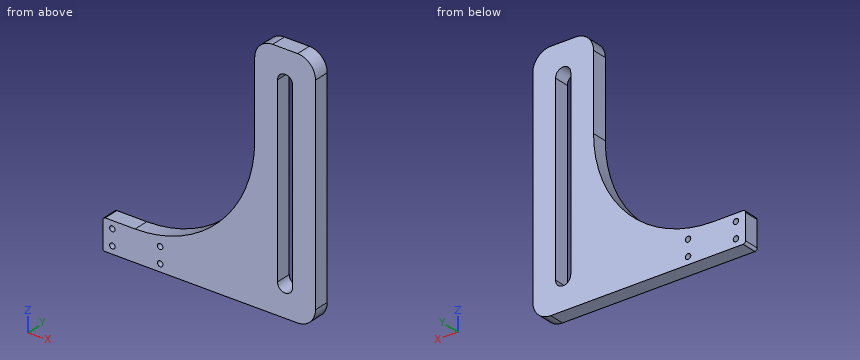
```python
from build123d import *

# Parameters (mm, degrees)
SKETCH1_R           = 1.1303
BOSS_EXTRUDE2_DEPTH = 6.35
FILLET1_R           = 1
FILLET2_R           = 7.5


with BuildPart() as part:
    # Sketch1 → Boss-Extrude2 (new body)
    with BuildSketch(Plane(origin=(0, 0, 0), x_dir=(1, 0, 0), z_dir=(0, 1, 0))):
        with BuildLine():
            Line((-12.7, 50.8), (-76.2, 50.8))
            Line((-76.2, 50.8), (-76.2, 38.1))
            Line((-76.2, 38.1), (-62.7, 38.1))
            ThreePointArc((-62.7, 38.1), (-27.344660941, 23.455339059), (-12.7, -11.9))
            Line((-12.7, -11.9), (-12.7, -50.8))
            Line((-12.7, -50.8), (12.7, -50.8))
            Line((12.7, -50.8), (12.7, 50.8))
            Line((12.7, 50.8), (-12.7, 50.8))
        make_face()
        with Locations(Location((-72.2, 47.7, 0), (0, 0, 270))):
            Circle(SKETCH1_R, mode=Mode.SUBTRACT)
        with Locations(Location((-72.2, 41.2, 0), (0, 0, 270))):
            Circle(SKETCH1_R, mode=Mode.SUBTRACT)
        with Locations(Location((-52.2, 47.7, 0), (0, 0, 270))):
            Circle(SKETCH1_R, mode=Mode.SUBTRACT)
        with Locations(Location((-52.2, 41.2, 0), (0, 0, 270))):
            Circle(SKETCH1_R, mode=Mode.SUBTRACT)
        with BuildLine():
            Line((-3.175, -38.1), (-3.175, 38.1))
            ThreePointArc((-3.175, 38.1), (0, 41.275), (3.175, 38.1))
            Line((3.175, 38.1), (3.175, -38.1))
            ThreePointArc((3.175, -38.1), (0, -41.275), (-3.175, -38.1))
        make_face(mode=Mode.SUBTRACT)
    extrude(amount=BOSS_EXTRUDE2_DEPTH)

    # Fillet1
    fillet1_edges = [part.edges().sort_by_distance(p)[0] for p in [
        (-76.2, 3.175, -38.1),
        (-76.2, 3.175, -50.8),
    ]]
    fillet(fillet1_edges, radius=FILLET1_R)

    # Fillet2
    fillet2_edges = [part.edges().sort_by_distance(p)[0] for p in [
        (12.7, 3.175, 50.8),
        (-12.7, 3.175, 50.8),
        (12.7, 3.175, -50.8),
    ]]
    fillet(fillet2_edges, radius=FILLET2_R)


solid = part.part
```
Model file for the job. Use its own axes, mm. Give positions to 0.01 mm unless a question says otherwise; leave off trailing zeros. Order: outer loops, then holes, each group sorted by start corner. A loop starts at its lowest first (then second) coordinate and runs counter-clockwise, first axis right, second up.
1) Pin check, flat tips, straight feed: pin 1 (1.5 mm diameter, centred on x = -30.5, y = 3, fed in from +Z); pin 2 (1.9 mm diameter, centred on y = 2, z = -7, fed in from -X); pin 3 (2 mm diameter, centred on y = 3, z = 22.5, fed in from -X). Stop position of each tip, or through.
2) Saw through at B-B, the plane x = -52.2. Write the cut outline in (y, z), then the cut area to 3 significant figures.
3) Wall check: probe 1 along Z at (x, y) = (-72.2, 5); probe 2 along X at (y, z) = (3, 33) (3 decimals); probe 3 along Z at (x, y) = (-52, 5). Give the ranges that are in metal, low to high.
4) Saw through at C-C, the plane y = 2. Write the cut outline in (x, z) (3 decimals), then the cut area to 3 significant figures.
5) Saw through at A-A, the plane z = -22. Write the cut outline in (x, y) (3 decimals), then the cut area to 3 significant figures.
6) Saw through at D-D, the plane z = -47.7. Write the cut outline in (x, y).
Computed:
1. pin 1: stops at z = -25.71
1. pin 2: stops at x = -16.81
1. pin 3: stops at x = -12.7
2. outline: (0, -50.8) - (6.35, -50.8) - (6.35, -48.83) - (0, -48.83) - close; (0, -46.57) - (6.35, -46.57) - (6.35, -42.33) - (0, -42.33) - close; (0, -40.07) - (6.35, -40.07) - (6.35, -36.99) - (0, -36.99) - close
2. area: 59.0 mm2
3. probe 1: z = -50.8 to -48.83, -46.57 to -42.33, -40.07 to -38.1
3. probe 2: x = -12.7 to -3.175, 3.175 to 12.7
3. probe 3: z = -50.8 to -48.81, -46.59 to -42.31, -40.09 to -36.94
4. outline: (-76.2, -49.8) arc R1 ccw to (-75.2, -50.8) - (5.2, -50.8) arc R7.5 ccw to (12.7, -43.3) - (12.7, 43.3) arc R7.5 ccw to (5.2, 50.8) - (-5.2, 50.8) arc R7.5 ccw to (-12.7, 43.3) - (-12.7, 11.9) arc R50 cw to (-62.7, -38.1) - (-75.2, -38.1) arc R1 ccw to (-76.2, -39.1) - close; hole circle Ø2.261 at (-72.2, -47.7); hole circle Ø2.261 at (-72.2, -41.2); hole circle Ø2.261 at (-52.2, -47.7); hole circle Ø2.261 at (-52.2, -41.2); hole (-3.175, -38.1) arc R3.175 ccw to (3.175, -38.1) - (3.175, 38.1) arc R3.175 ccw to (-3.175, 38.1) - close
4. area: 3,360 mm2
5. outline: (-25.947, 0) - (-3.175, 0) - (-3.175, 6.35) - (-25.947, 6.35) - close; (3.175, 0) - (12.7, 0) - (12.7, 6.35) - (3.175, 6.35) - close
5. area: 205 mm2
6. outline: (-76.2, 0) - (-73.33, 0) - (-73.33, 6.35) - (-76.2, 6.35) - close; (-71.07, 0) - (-53.33, 0) - (-53.33, 6.35) - (-71.07, 6.35) - close; (-51.07, 0) - (11.27, 0) - (11.27, 6.35) - (-51.07, 6.35) - close
